Work out the finished part from the listing and answer in its coordinate system (mm). Face numbers are marked on the shaded views. A direction names the side the tool comes from. Round coordinates to 2 decimals unless told otherwise and drop trailing zeros. Loops run counter-clockwise (first coordinate to the right, second up) from the corner with the lowest first, then second, coordinate; pieces in that order, holes last. Notation, with made-up numbers: (75.5, -17.5) - (114.5, -17.5) arc R12 ccw to (114.5, -0.5) - close; hole circle Ø1 at (18.25, 71.25). An arc over 180 degrees is marked (long way). Answer as CSV lines item,"result". Start each with the question number.
```python
from build123d import *

# Parameters (mm, degrees)
SKETCH1_W           = 40
SKETCH1_H           = 20
BOSS_EXTRUDE1_DEPTH = 28
SKETCH2_W           = 54.5
SKETCH2_H           = 20
BOSS_EXTRUDE2_DEPTH = 3
SKETCH3_W           = 40
SKETCH3_H           = 20
BOSS_EXTRUDE3_DEPTH = 9.5
SKETCH4_R           = 2.925
BOSS_EXTRUDE4_DEPTH = 5
SKETCH5_R           = 2.5
CUT_EXTRUDE1_DEPTH  = 3
BOSS_EXTRUDE5_START = -10
BOSS_EXTRUDE5_DEPTH = 0.75


with BuildPart() as part:
    # Sketch1 → Boss-Extrude1 (new body)
    with BuildSketch(Plane(origin=(0, 0, 0), x_dir=(1, 0, 0), z_dir=(0, 1, 0))):
        Rectangle(SKETCH1_W, SKETCH1_H)
    extrude(amount=-BOSS_EXTRUDE1_DEPTH)

    # Sketch2 → Boss-Extrude2 (add)
    with BuildSketch(Plane(origin=(0, 0, 0), x_dir=(1, 0, 0), z_dir=(0, 1, 0))):
        Rectangle(SKETCH2_W, SKETCH2_H)
    extrude(amount=BOSS_EXTRUDE2_DEPTH)

    # Sketch3 → Boss-Extrude3 (add)
    with BuildSketch(Plane(origin=(0, 3, 0), x_dir=(1, 0, 0), z_dir=(0, 1, 0))):
        Rectangle(SKETCH3_W, SKETCH3_H)
    extrude(amount=BOSS_EXTRUDE3_DEPTH)

    # Sketch4 → Boss-Extrude4 (add)
    with BuildSketch(Plane(origin=(0, 12.5, 0), x_dir=(1, 0, 0), z_dir=(0, 1, 0))):
        with Locations(Location((10, 0, 0), (0, 0, 270))):
            Circle(SKETCH4_R)
    extrude(amount=BOSS_EXTRUDE4_DEPTH)

    # Sketch5 → Cut-Extrude1 (cut)
    with BuildSketch(Plane(origin=(0, 3, 0), x_dir=(1, 0, 0), z_dir=(0, 1, 0))):
        with Locations((25.15, -6)):
            Circle(SKETCH5_R)
        with Locations((25.15, 6)):
            Circle(SKETCH5_R)
        with Locations((-25.15, -6)):
            Circle(SKETCH5_R)
        with Locations((-25.15, 6)):
            Circle(SKETCH5_R)
    extrude(amount=-CUT_EXTRUDE1_DEPTH, mode=Mode.SUBTRACT)

    # Sketch6 → Boss-Extrude5 (add, symmetric)
    with BuildSketch(Plane(origin=(0, 0, -10), x_dir=(-1, 0, 0), z_dir=(0, 0, -1)).offset(BOSS_EXTRUDE5_START)):
        Polygon((-20, 3), (-20, 4.9), (-21, 4.9), (-26.25, 3.5), (-26.25, 3), align=None)
    boss_extrude5 = extrude(amount=BOSS_EXTRUDE5_DEPTH, both=True)

    # Mirror1: Boss-Extrude5 across plane
    add(boss_extrude5.mirror(Plane(origin=(0, 0, 0), x_dir=(0, 0, 1), z_dir=(1, 0, 0))))


solid = part.part
```
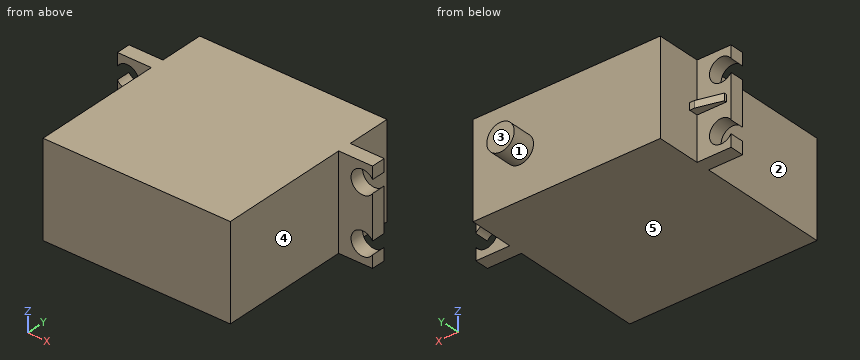
Item 1: Section D-D, the plane x = -25.15 is taken. Give the vertices of the cut face in (y, z), and give its area (3 significant figures).
Item 2: Section C-C, the plane z = 6 is taken. Give the vertices of the cut face in (x, y).
Item 3: Find the intervals of material crossed by L1, parallel to Z at x = 25.15, y = 0.85; L2, parallel to Y at x = -23, z = -3; L3, parallel to X at y = 12, z = 8.75, in increasing order.
Item 4: Which of the six approach directions +Z, -Z, +X, -X, +Y, -Y give full straight-line access (tool end or side, diameter ignored) to the marked faces 1, 2, 3, 4 and 5?
Item 5: Section B-B, the plane x = 10 is taken. Give the vertices of the cut face in (y, z) (3 decimals).
Item 6: Flat-ended cylindrical pins translate along their axes: pin 1 Ø1.5 at (y, z) = (12.5, 7) entering from -X; pin 2 Ø8 at (x, z) = (25.15, 6) entering from -Y; pin 3 Ø5 at (y, z) = (10, 0.5) entering from +X. Find the tip coordinate at first contact, or state that the pin passes through.
Item 7: Section A-A, the plane y = 2 is taken. Give the vertices of the cut face in (x, z), and give its area (3 significant figures).
Answer:
1,outline,"(0, -10) - (3, -10) - (3, -8.5) - (0, -8.5) - close; (0, -3.5) - (3, -3.5) - (3, -0.75) - (3.79, -0.75) - (3.79, 0.75) - (3, 0.75) - (3, 3.5) - (0, 3.5) - close; (0, 8.5) - (3, 8.5) - (3, 10) - (0, 10) - close"
1,area,"31.2 mm²"
2,outline,"(-22.65, 0) - (-20, 0) - (-20, -28) - (20, -28) - (20, 0) - (22.65, 0) - (22.65, 3) - (20, 3) - (20, 12.5) - (-20, 12.5) - (-20, 3) - (-22.65, 3) - close"
3,L1,"z = -10 to -8.5, -3.5 to 3.5, 8.5 to 10"
3,L2,"y = 0 to 3"
3,L3,"x = -20 to 20"
4,face 1,"+Y"
4,face 2,"+Z, -Z, -X, -Y"
4,face 3,"+Z, -Z, +X, -X, +Y"
4,face 4,"+Z, -Z, +X, -Y"
4,face 5,"-Z, +X, -X, +Y, -Y"
5,outline,"(-28, -10) - (12.5, -10) - (12.5, -2.925) - (17.5, -2.925) - (17.5, 2.925) - (12.5, 2.925) - (12.5, 10) - (-28, 10) - close"
6,pin 1,"stops at x = -20"
6,pin 2,"stops at y = 0"
6,pin 3,"stops at x = 20"
7,outline,"(-27.25, -10) - (27.25, -10) - (27.25, -7.36) arc R2.5 cw (long way) to (27.25, -4.64) - (27.25, 4.64) arc R2.5 cw (long way) to (27.25, 7.36) - (27.25, 10) - (-27.25, 10) - (-27.25, 7.36) arc R2.5 cw (long way) to (-27.25, 4.64) - (-27.25, -4.64) arc R2.5 cw (long way) to (-27.25, -7.36) - close"
7,area,"1,010 mm²"
